Input: part model. Units: mm. Frame: model coordinates. Face numbers are marked on the shaded views. A direction names the side the tool comes from. Round coordinates to 2 decimals unless told otherwise and drop trailing zeros. Loops run counter-clockwise (first coordinate to the right, second up) from the corner with the lowest first, then second, coordinate; pieces in that order, holes last.
1) First-contact query: pin 1 (10 mm diameter, centred on x = 2.5, y = -6, fed in from +Z); pin 2 (8 mm diameter, centred on x = -9, y = -19.5, fed in from +Z); pin 3 (3 mm diameter, centred on x = -3.5, z = 2.5, fed in from -Y). Flat tips, straight axial feed; report the tip coordinate or a pass-through.
2) Access query for the marked faces 1, 2 and 3. Directions: +Z, -Z, +X, -X, +Y, -Y. A direction counts if a zero-diameter tool reaches every point of the face in a straight line with its end or side. Return the directions, or none.
3) Draft query along X for the marked faces 4, 5 and 6. Return one class per face: pulls with the +X half, pulls with the -X half, needs draft (parallel to the pull), parting line crosses it, or undercut.
4) Section B-B, the plane y = -3. Return loops of the section in (x, z), and give its area (3 significant figures).
5) Section A-A, the plane z = 0.25. Return loops of the section in (x, y), and give its area (3 significant figures).
6) Section D-D, the plane z = 3.75. Return loops of the section in (x, y).
7) Section C-C, the plane x = -1.5. Return loops of the section in (y, z), and give its area (3 significant figures).
8) Ray query, line 1 along Z through (x, y) = (-3.25, -8.25); line 2 along Y through (x, z) = (-11.25, 5.5); line 3 along X through (y, z) = (-4.25, -0.5). Return the intervals inside material, ascending.
from build123d import *

# Parameters (mm, degrees)
F0_W     = 25.4
F0_H     = 12.7
F1_DEPTH = 25.4
F3_DEPTH = 7.62
F5_DEPTH = 7.62
F6_R     = 8.47557
F7_DEPTH = 25.4


with BuildPart() as f1:
    # F0 (on Front) → F1 (new body)
    with BuildSketch(Plane.XZ):
        Rectangle(F0_W, F0_H)
    extrude(amount=F1_DEPTH)

    # F2 (on face) → F3 (cut)
    with BuildSketch(Plane.XY.offset(6.35)):
        Polygon((-6.431355, 0), (-9.439249, -25.4), (-1.919514, -25.4), (1.08838, 0), align=None)
    extrude(amount=-F3_DEPTH, mode=Mode.SUBTRACT)

    # F4 (on face) → F5 (cut)
    with BuildSketch(Plane.XY.offset(6.35)):
        Polygon((-1.919514, -25.4), (5.390243, -25.4), (8.398137, 0), (1.08838, 0), align=None)
    extrude(amount=-F5_DEPTH, mode=Mode.SUBTRACT)

    # F6 (on face) → F7 (cut)
    with BuildSketch(Plane.YZ.offset(12.7)):
        with Locations((-12.7, 6.35)):
            Circle(F6_R)
    extrude(amount=-F7_DEPTH, mode=Mode.SUBTRACT)


solid = f1.part
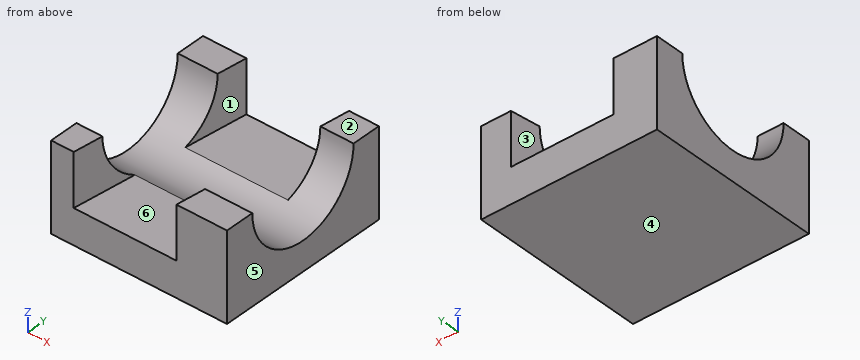
Final values:
1. pin 1: stops at z = -1.27
1. pin 2: stops at z = 6.35
1. pin 3: passes through
2. face 1: +Z, -Y
2. face 2: +Z, +X, -X, +Y, -Y
2. face 3: +Z, +Y
3. face 4: needs draft
3. face 5: pulls with the +X half
3. face 6: undercut
4. outline: (-12.7, -6.35) - (12.7, -6.35) - (12.7, 6.35) - (8.04, 6.35) - (8.04, -1.27) - (-6.79, -1.27) - (-6.79, 6.35) - (-12.7, 6.35) - close
4. area: 210 mm2
5. outline: (-12.7, -25.4) - (-9.44, -25.4) - (-8.63, -18.58) - (-12.7, -18.58) - close; (-12.7, -6.82) - (-7.24, -6.82) - (-6.43, 0) - (-12.7, 0) - close; (5.39, -25.4) - (12.7, -25.4) - (12.7, -18.58) - (6.2, -18.58) - close; (7.59, -6.82) - (12.7, -6.82) - (12.7, 0) - (8.4, 0) - close
5. area: 144 mm2
6. outline: (-12.7, -25.4) - (-9.44, -25.4) - (-8.89, -20.77) - (-12.7, -20.77) - close; (-12.7, -4.63) - (-6.98, -4.63) - (-6.43, 0) - (-12.7, 0) - close; (5.39, -25.4) - (12.7, -25.4) - (12.7, -20.77) - (5.94, -20.77) - close; (7.85, -4.63) - (12.7, -4.63) - (12.7, 0) - (8.4, 0) - close
7. outline: (-25.4, -6.35) - (0, -6.35) - (0, -1.27) - (-8.99, -1.27) arc R8.48 cw to (-16.41, -1.27) - (-25.4, -1.27) - close
7. area: 125 mm2
8. line 1: z = -6.35 to -1.27
8. line 2: y = -25.4 to -21.13, -4.27 to 0
8. line 3: x = -12.7 to -6.93, 7.89 to 12.7
